Answer from the drawing. Dimensions are ordinates in mm from the lowest x, y and z of the part. A direction names the side the tool comes from. Give positions to 0.01 mm unless a question says otherwise; leave off trailing zeros. Write each loop counter-clockwise with the first axis right and the second up, starting at its lowest first coordinate (ties: lowest second). Pieces come first, ordered by that corner, then holes. Notation, with made-up numbers: M -19,35.5 L -6,35.5 A13 cw -6,44.5 Z; hole C 35,85.5 d2. An arc over 180 degrees is marked long. Put each result on its own line as item: value.
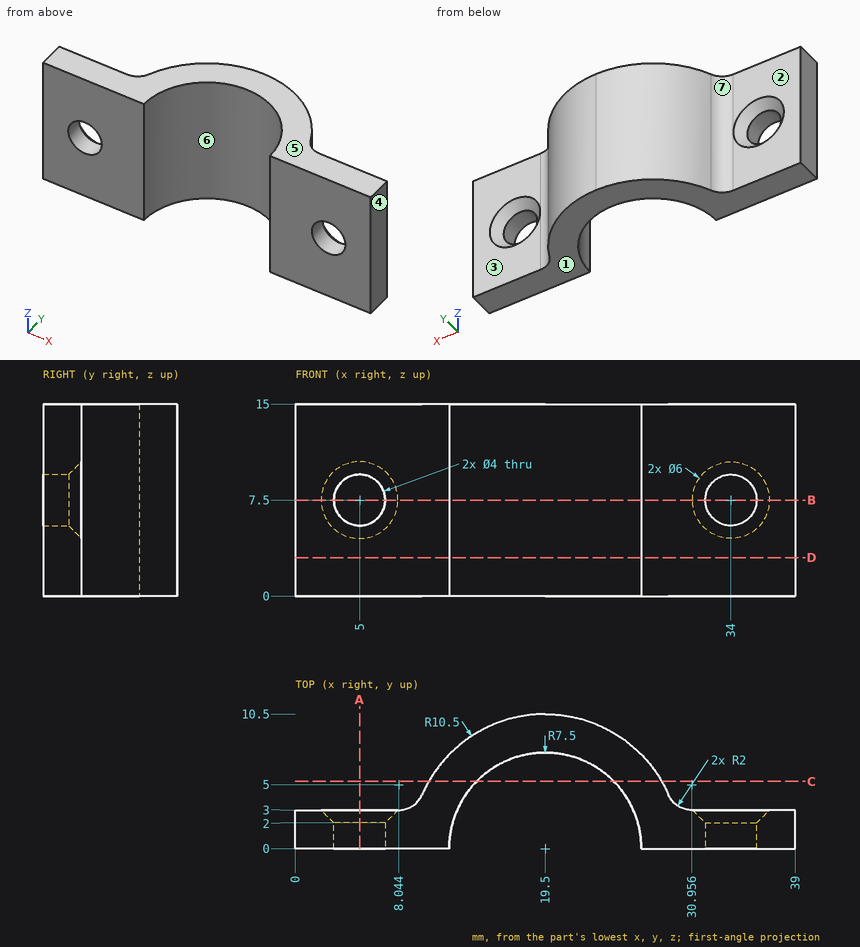
(1) For a pull along X with two mould halves and no side action, classify the marked faces 4, 5, 6 and 7 as +X half, -X half, draft (parallel to the pull), parting line (faces both ways), or undercut.
Result:
face 4: +X half
face 5: draft
face 6: undercut
face 7: -X half
(2) Section A-A on x = 5 is taken. Determine the outline of the cut face in (y, z), and give its area (3 significant figures).
Result:
outline: M 0,0 L 3,0 L 3,4.5 L 2,5.5 L 0,5.5 Z; M 0,9.5 L 2,9.5 L 3,10.5 L 3,15 L 0,15 Z
area: 32.0 mm²
(3) Section B-B on z = 7.5 is taken. Determine the outline of the cut face in (x, y).
Result:
outline: M 0,0 L 3,0 L 3,2 L 2,3 L 0,3 Z; M 7,0 L 12,0 A7.5 cw 27,0 L 32,0 L 32,2 L 31,3 L 30.96,3 A2 cw 29.12,4.2 A10.5 ccw 19.5,10.5 A10.5 ccw 9.88,4.2 A2 cw 8.04,3 L 8,3 L 7,2 Z; M 36,0 L 39,0 L 39,3 L 37,3 L 36,2 Z
(4) Which of the six approach directions +Z, -Z, +X, -X, +Y, -Y give full straight-line access (tool end or side, diameter ignored) to the marked faces 1, 2 and 3?
Result:
face 1: -Z, +X, -X, +Y, -Y
face 2: +Z, -Z, -X, +Y
face 3: +Z, -Z, +X, +Y
(5) Section D-D on z = 3 is taken. Determine the outline of the cut face in (x, y).
Result:
outline: M 0,0 L 12,0 A7.5 cw 27,0 L 39,0 L 39,3 L 30.96,3 A2 cw 29.12,4.2 A10.5 ccw 19.5,10.5 A10.5 ccw 9.88,4.2 A2 cw 8.04,3 L 0,3 Z
(6) Section C-C on y = 5.25 is taken. Determine the outline of the cut face in (x, z).
Result:
outline: M 10.41,0 L 14.14,0 L 14.14,15 L 10.41,15 Z; M 24.86,0 L 28.59,0 L 28.59,15 L 24.86,15 Z
(7) Given pin 1 Ø4 at (x, z) = (4.5, 11) entering from +Y; pin 2 Ø1 at (x, z) = (11.5, 10.5) entering from +Y; pin 3 Ø1 at (y, z) = (5, 2) entering from -X, each flat-ended and moving along its own axis, determine where each tip first touches the part or whether it passes through.
Result:
pin 1: stops at y = 3
pin 2: stops at y = 7.35
pin 3: stops at x = 10.01
(8) Straight lines are drawn through the part: line 1 along Z through (x, y) = (5, 1); line 2 along X through (y, z) = (2, 14); line 3 along Y through (x, z) = (36, 5). For each, find the intervals that lie inside material, in ascending order. Write a range as from..to.
Result:
line 1: z = 0..5.5, 9.5..15
line 2: x = 0..12.27, 26.73..39
line 3: y = 0..3
